from build123d import *

# Parameters (mm, degrees)
BOSS_EXTRUDE1_DEPTH      = 1.5
BOSS_EXTRUDE1_DEPTH_BACK = 1.5
SKETCH2_W                = 12.59
SKETCH2_H                = 23.03
CUT_EXTRUDE1_DEPTH       = 3
SKETCH3_W                = 12.59
SKETCH3_H                = 23.03
CUT_EXTRUDE2_DEPTH       = 3
CUT_EXTRUDE3_DEPTH       = 3
CUT_EXTRUDE4_DEPTH       = 3
CUT_EXTRUDE5_DEPTH       = 3
CUT_EXTRUDE6_DEPTH       = 3
SKETCH8_R                = 9.96
CUT_EXTRUDE7_DEPTH       = 3
SKETCH9_R                = 1.59
CUT_EXTRUDE8_DEPTH       = 3
SKETCH10_R               = 1.59
CUT_EXTRUDE9_DEPTH       = 3


with BuildPart() as part:
    # Sketch1 → Boss-Extrude1 (new, two sides: drawn at the far end of the back side and taken through both)
    with BuildSketch(Plane.XY.offset(-BOSS_EXTRUDE1_DEPTH_BACK)):
        with BuildLine():
            Line((98.253494636, -20.43499635), (104.23425822, -10.0760127))
            Line((104.23425822, -10.0760127), (113.064881921, -7.709853588))
            ThreePointArc((113.064881921, -7.709853588), (121.722656845, -5.725791507), (127.769789966, 0.780032806))
            Line((127.769789966, 0.780032806), (134.234253695, 7.24450012))
            Line((134.234253695, 7.24450012), (146.195780864, 7.24450012))
            Line((146.195780864, 7.24450012), (152.660249109, 0.78003546))
            ThreePointArc((152.660249109, 0.78003546), (158.707381887, -5.725786628), (167.365155021, -7.709848177))
            Line((167.365155021, -7.709848177), (176.195776859, -10.076007288))
            Line((176.195776859, -10.076007288), (182.176542181, -20.434992087))
            Line((182.176542181, -20.434992087), (179.810382355, -29.265616594))
            ThreePointArc((179.810382355, -29.265616594), (177.199740829, -37.75550103), (179.810382355, -46.245385467))
            Line((179.810382355, -46.245385467), (182.176541113, -55.07600785))
            Line((182.176541113, -55.07600785), (176.195778722, -65.434989434))
            Line((176.195778722, -65.434989434), (167.365155827, -67.801148329))
            ThreePointArc((167.365155827, -67.801148329), (158.707382848, -69.785210553), (152.660250576, -76.291033111))
            Line((152.660250576, -76.291033111), (146.195785916, -82.755501356))
            Line((146.195785916, -82.755501356), (134.234258747, -82.755501356))
            Line((134.234258747, -82.755501356), (127.769791434, -76.291037627))
            ThreePointArc((127.769791434, -76.291037627), (121.722657806, -69.785213784), (113.064882728, -67.801152377))
            Line((113.064882728, -67.801152377), (104.23425822, -65.434992551))
            Line((104.23425822, -65.434992551), (98.253494636, -55.076010763))
            Line((98.253494636, -55.076010763), (100.619653747, -46.245388924))
            ThreePointArc((100.619653747, -46.245388924), (103.230295273, -37.755504488), (100.619653747, -29.265620052))
            Line((100.619653747, -29.265620052), (98.253494636, -20.43499635))
        make_face()
    extrude(amount=BOSS_EXTRUDE1_DEPTH + BOSS_EXTRUDE1_DEPTH_BACK)

    # Sketch2 → Cut-Extrude1 (cut)
    with BuildSketch(Plane.XY.offset(1.5)):
        with Locations((139.900780864, -9.59049988)):
            Rectangle(SKETCH2_W, SKETCH2_H)
    extrude(amount=-CUT_EXTRUDE1_DEPTH, mode=Mode.SUBTRACT)

    # Sketch3 → Cut-Extrude2 (cut)
    with BuildSketch(Plane.XY.offset(1.5)):
        with Locations((140.529262159, -65.920502947)):
            Rectangle(SKETCH3_W, SKETCH3_H)
    extrude(amount=-CUT_EXTRUDE2_DEPTH, mode=Mode.SUBTRACT)

    # Sketch4 → Cut-Extrude3 (cut)
    with BuildSketch(Plane.XY.offset(1.5)):
        Polygon((171.588522223, -12.736008176), (151.64395758, -24.251013064), (157.624720423, -34.609993567), (177.569285268, -23.094993214), align=None)
    extrude(amount=-CUT_EXTRUDE3_DEPTH, mode=Mode.SUBTRACT)

    # Sketch5 → Cut-Extrude4 (cut)
    with BuildSketch(Plane.XY.offset(1.5)):
        Polygon((102.86074998, -52.416011103), (122.80531503, -40.901011103), (128.786075877, -51.259992759), (108.841510828, -62.774992759), align=None)
    extrude(amount=-CUT_EXTRUDE4_DEPTH, mode=Mode.SUBTRACT)

    # Sketch6 → Cut-Extrude5 (cut)
    with BuildSketch(Plane.XY.offset(1.5)):
        Polygon((108.841512319, -12.736014517), (128.78607799, -24.25101344), (122.805317347, -34.609996033), (102.860751676, -23.094997111), align=None)
    extrude(amount=-CUT_EXTRUDE5_DEPTH, mode=Mode.SUBTRACT)

    # Sketch7 → Cut-Extrude6 (cut)
    with BuildSketch(Plane.XY.offset(1.5)):
        Polygon((151.643959507, -51.25999177), (171.588525178, -62.774990693), (177.569285821, -52.416008099), (157.62472015, -40.901009176), align=None)
    extrude(amount=-CUT_EXTRUDE6_DEPTH, mode=Mode.SUBTRACT)

    # Sketch8 → Cut-Extrude7 (cut)
    with BuildSketch(Plane.XY.offset(1.5)):
        with Locations((140.215021511, -37.755501414)):
            Circle(SKETCH8_R)
    extrude(amount=-CUT_EXTRUDE7_DEPTH, mode=Mode.SUBTRACT)

    # Sketch9 → Cut-Extrude8 (cut)
    with BuildSketch(Plane.XY.offset(1.5)):
        with Locations((127.717657389, -59.401568952)):
            Circle(SKETCH9_R)
    extrude(amount=-CUT_EXTRUDE8_DEPTH, mode=Mode.SUBTRACT)

    # Sketch10 → Cut-Extrude9 (cut)
    with BuildSketch(Plane.XY.offset(1.5)):
        with Locations((152.712382304, -16.10943146)):
            Circle(SKETCH10_R)
        with Locations((165.209740829, -37.75550103)):
            Circle(SKETCH10_R)
        with Locations((115.220295273, -37.75550103)):
            Circle(SKETCH10_R)
        with Locations((127.717654681, -16.10943146)):
            Circle(SKETCH10_R)
        with Locations((152.712382304, -59.40156591)):
            Circle(SKETCH10_R)
    extrude(amount=-CUT_EXTRUDE9_DEPTH, mode=Mode.SUBTRACT)


solid = part.part
Input: part model. Units: mm. Frame: model coordinates. A direction names the side the tool comes from. Coordinates: 2 decimals unless noted, no trailing zeros. Order: outer loops, then holes, each group sorted by start corner. A loop starts at its lowest first (then second) coordinate and runs counter-clockwise, first axis right, second up.
1. Contact query for a flat-ended pin moving along its axis: P1, Ø4, axis at x = 127.72, y = -59.4, coming from the +Z side. Output: stop coordinate, or through.
Checked values:
P1: stops at z = 1.5
2. Cut plane A-A, the plane x = 144.5. Return loops of the section in (y, z), plus the area to 3 significant figures.
Checked values:
outline: (-82.76, -1.5) - (-77.44, -1.5) - (-77.44, 1.5) - (-82.76, 1.5) - close; (-54.41, -1.5) - (-46.75, -1.5) - (-46.75, 1.5) - (-54.41, 1.5) - close; (-28.76, -1.5) - (-21.11, -1.5) - (-21.11, 1.5) - (-28.76, 1.5) - close; (1.92, -1.5) - (7.24, -1.5) - (7.24, 1.5) - (1.92, 1.5) - close
area: 77.9 mm2
3. Draft query along X for faces 1 (the cylindrical face through (103.23, -37.88, -0.02)), 2 (the flat face through (141, -27, -1.5)), 3 (the cylindrical face through (151.124, -16.04, 0.021)). Return one class per face: +X half, -X half, draft (parallel to the pull), parting line (faces both ways), or undercut.
Checked values:
face 1: -X half
face 2: draft
face 3: undercut
4. Cut plane D-D, the plane x = 106.5. Return loops of the section in (y, z), plus the area to 3 significant figures.
Checked values:
outline: (-66.04, -1.5) - (-58.72, -1.5) - (-58.72, 1.5) - (-66.04, 1.5) - close; (-50.31, -1.5) - (-25.2, -1.5) - (-25.2, 1.5) - (-50.31, 1.5) - close; (-16.79, -1.5) - (-9.47, -1.5) - (-9.47, 1.5) - (-16.79, 1.5) - close
area: 119 mm2
5. Cut plane C-C, the plane x = 121. Return loops of the section in (y, z).
Checked values:
outline: (-69.39, -1.5) - (-55.76, -1.5) - (-55.76, 1.5) - (-69.39, 1.5) - close; (-41.94, -1.5) - (-33.57, -1.5) - (-33.57, 1.5) - (-41.94, 1.5) - close; (-19.76, -1.5) - (-6.12, -1.5) - (-6.12, 1.5) - (-19.76, 1.5) - close
6. Ray query, line 1 along Y through (x, z) = (111, 0.1); line 2 along Y through (x, z) = (161, -0.4); line 3 along X through (y, z) = (-59.5, 0.8). Return the intervals inside material, ascending.
Checked values:
line 1: y = -67.25 to -61.53, -47.72 to -27.79, -13.98 to -8.26
line 2: y = -68.71 to -56.66, -42.85 to -32.66, -18.85 to -6.8
line 3: x = 100.81 to 106.95, 114.51 to 126.13, 129.3 to 134.23, 146.82 to 151.13, 154.3 to 165.92, 173.48 to 179.62
7. Access query for faces 4 (the flat face through (130.96, 3.97, -0.02)), 5 (the flat face through (146.824, -66, 0)), 6 (the flat face through (181.01, -24.79, -0.02)). Directions: +Z, -Z, +X, -X, +Y, -Y. A direction counts if a zero-diameter tool reaches every point of the face in a straight line with its end or side. Return the directions, or none.
Checked values:
face 4: +Z, -Z, -X, +Y
face 5: +Z, -Z
face 6: +Z, -Z, +X
8. Cut plane B-B, the plane y = -42. Return loops of the section in (x, z), plus the area to 3 significant figures.
Checked values:
outline: (102.62, -1.5) - (120.9, -1.5) - (120.9, 1.5) - (102.62, 1.5) - close; (123.44, -1.5) - (131.2, -1.5) - (131.2, 1.5) - (123.44, 1.5) - close; (149.23, -1.5) - (156.99, -1.5) - (156.99, 1.5) - (149.23, 1.5) - close; (159.53, -1.5) - (177.81, -1.5) - (177.81, 1.5) - (159.53, 1.5) - close
area: 156 mm2
